Autodesk Inventor part; units mm, degrees
ref_plane "Work Plane1" through (0, 0.77, 0) normal (0, -1, 0) x (1, 0, 0)
ref_plane "YZ Plane" through (0, 0, 0) normal (1, 0, 0) x (0, 1, 0)
ref_plane "XZ Plane" through (0, 0, 0) normal (0, 1, 0) x (-1, 0, 0)
sketch "Sketch1" plane through (0, 0, 0) normal (0, 1, 0) x (-1, 0, 0)
  line L0 (0, 0) -> (25.5, 0)
  line L1 (25.5, 0) -> (25.5, -17.7)
  line L2 (25.5, -17.7) -> (0, -17.7)
  line L3 (0, -17.7) -> (0, 0)
  dimension "d0" = 25.5
  dimension "d1" = 17.7
extrude "Extrusion1" add sketch "Sketch1" along normal blind 1.54
sketch "Sketch2" plane through (0, 1.54, 0) normal (0, 1, 0) x (1, 0, 0)
  line L0 (-25.5, 0) -> (0, 0)
  line L1 (0, 0) -> (-2.5, 0)
  line L2 (-2.5, 0) -> (-2.5, 1.25)
  line L3 (-2.5, 2.5) -> (0, 2.5)
  line L4 (0, 2.5) -> (0, 0)
  circle A0 centre (-2.5, 2.5) radius 1.25
  line L5 (0, 17.7) -> (-25.5, 17.7)
  line L6 (0, 0) -> (0, 17.7)
  line L7 (0, 17.7) -> (0, 8.85)
  line L8 (0, 0) -> (0, 17.7)
  line L9 (0, 8.85) -> (-1.25, 8.85)
  line L10 (-25.5, 17.7) -> (0, 17.7)
  line L11 (-12.75, 17.7) -> (-12.75, 15.5963)
  circle A1 centre (-23, 2.5) radius 1.25
  circle A2 centre (-2.5, 15.2) radius 1.25
  circle A3 centre (-23, 15.2) radius 1.25
  dimension "d6" = 2.5
  dimension "d4" = 2.5
  dimension "d5" = 2.5
extrude "Extrusion2" cut sketch "Sketch2" against normal blind 1.54 contours A0 | A1 | A2 | A3
sketch "Sketch3" plane through (0, 0, 0) normal (1, 0, 0) x (0, 0, -1)
  line L0 (0, 0) -> (0, 1.54)
  line L1 (17.7, 0) -> (17.7, 1.54)
  line L2 (0, 0) -> (17.7, 0)
  line L3 (0, 0) -> (17.7, 0)
  line L4 (8.85, 0) -> (11.85, 0)
  line L5 (11.85, 0) -> (11.85, 4.5)
  line L6 (11.85, 4.5) -> (5.85, 4.5)
  line L7 (5.85, 4.5) -> (5.85, 0)
  line L8 (5.85, 4.5) -> (11.85, 4.5)
  line L9 (11.85, 4.5) -> (11.85, 0)
  line L10 (11.85, 0) -> (5.85, 0)
  line L11 (5.85, 0) -> (5.85, 4.5)
  dimension "d9" = 3
  dimension "d10" = 4.5
  dimension "d11" = 6
extrude "Extrusion3" add sketch "Sketch3" against normal blind 25.5
sketch "Sketch4" plane through (0, 0, 0) normal (0, -1, 0) x (1, 0, 0)
  line L0 (0, -17.7) -> (-25.5, -17.7)
  line L1 (-9.0744, -17.7) -> (-16.5446, -17.7)
  line L2 (-16.5446, -17.7) -> (-16.5446, -15.2098)
  line L3 (-16.5446, -15.2098) -> (-9.0744, -15.2098)
  line L4 (-9.0744, -15.2098) -> (-9.0744, -17.7)
  point P0 (0, 0)
extrude "Extrusion4" add sketch "Sketch4" along normal blind 1.5
ref_plane "Work Plane1" through (0, 0.77, 0) normal (0, -1, 0) x (1, 0, 0)
mirror "Mirror1" about plane through (0, 0.77, 0) normal (0, -1, 0) of "Extrusion4"
properties part number "IMU-mpu6050"
The listing builds one solid part. Answer for the finished solid, in the listing's coordinates (mm). A direction names the side the tool comes from. Give positions to 0.01 mm unless a question says otherwise; leave off trailing zeros. Order: outer loops, then holes, each group sorted by start corner. A loop starts at its lowest first (then second) coordinate and runs counter-clockwise, first axis right, second up.
Item 1: The part is cut by section A-A, the plane z = -2.5. Give the vertices of the cut face in (x, y).
From the geometry:
outline: (-25.5, 0) - (-24.25, 0) - (-24.25, 1.54) - (-25.5, 1.54) - close; (-21.75, 0) - (-3.75, 0) - (-3.75, 1.54) - (-21.75, 1.54) - close; (-1.25, 0) - (0, 0) - (0, 1.54) - (-1.25, 1.54) - close
Item 2: Given pin 1 Ø2 at (x, z) = (-22.5, -6) entering from -Y; pin 2 Ø1.6 at (x, y) = (-12.5, -1) entering from +Z; pin 3 Ø0.9 at (x, y) = (-19, 3.5) entering from -Z; pin 4 Ø2 at (x, z) = (-2.5, -2.5) entering from +Y, each flat-ended and moving along its own axis, determine where each tip first touches the part or whether it passes through.
From the geometry:
pin 1: stops at y = 0
pin 2: stops at z = -15.21
pin 3: stops at z = -11.85
pin 4: passes through
Item 3: Which of the six approach directions +Z, -Z, +X, -X, +Y, -Y give full straight-line access (tool end or side, diameter ignored) to faces 1 (the face through (-13, 3, -5.85)), 2 (the face through (-13, 3.04, -16)), 3 (the face through (-9.074, 2, -16))?
From the geometry:
face 1: +Z, +X, -X, +Y
face 2: -Z, +X, -X, +Y
face 3: -Z, +X, +Y
Item 4: The part is cut by section B-B, the plane x = -2.5. Give the vertices of the cut face in (y, z), and give its area (3 significant figures).
From the geometry:
outline: (0, -17.7) - (1.54, -17.7) - (1.54, -16.45) - (0, -16.45) - close; (0, -13.95) - (1.54, -13.95) - (1.54, -11.85) - (4.5, -11.85) - (4.5, -5.85) - (1.54, -5.85) - (1.54, -3.75) - (0, -3.75) - close; (0, -1.25) - (1.54, -1.25) - (1.54, 0) - (0, 0) - close
area: 37.3 mm2
Item 5: The part is cut by section D-D, the plane x = -10.75. Give the vertices of the cut face in (y, z).
From the geometry:
outline: (-1.5, -17.7) - (3.04, -17.7) - (3.04, -15.21) - (1.54, -15.21) - (1.54, -11.85) - (4.5, -11.85) - (4.5, -5.85) - (1.54, -5.85) - (1.54, 0) - (0, 0) - (0, -15.21) - (-1.5, -15.21) - close
Item 6: The part is cut by section C-C, the plane y = 1.8. Give the vertices of the cut face in (x, z), and give its area (3 significant figures).
From the geometry:
outline: (-25.5, -11.85) - (0, -11.85) - (0, -5.85) - (-25.5, -5.85) - close; (-16.54, -17.7) - (-9.07, -17.7) - (-9.07, -15.21) - (-16.54, -15.21) - close
area: 172 mm2
Item 7: Find the intervals of material crossed by probe 1 along X at (y, z) = (1.05, -15.2); probe 2 along Z at (x, y) = (-23, 0.35); probe 3 along Z at (x, y) = (-22.25, 0.55), in increasing order.
From the geometry:
probe 1: x = -25.5 to -24.25, -21.75 to -3.75, -1.25 to 0
probe 2: z = -17.7 to -16.45, -13.95 to -3.75, -1.25 to 0
probe 3: z = -17.7 to -16.2, -14.2 to -3.5, -1.5 to 0
Item 8: For a pull along X with two mould halves and no side action, classify faces 4 (the face through (-13, 1.54, -15)), 5 (the face through (-1.828, 0.781, -16.254)), 6 (the face through (-16.545, -1, -16)), 7 (the face through (-1.31, 0.78, -2.88)) as pulls with the +X half, pulls with the -X half, needs draft (parallel to the pull), parting line crosses it, or undercut.
From the geometry:
face 4: needs draft
face 5: undercut
face 6: pulls with the -X half
face 7: undercut
